```python
from build123d import *

# Parameters (mm, degrees)
F0_R     = 50.8
F1_DEPTH = 635
F2_W     = 50.8
F2_H     = 50.8
F3_DEPTH = 76.2
F4_R     = 19.05


with BuildPart() as f1:
    # F0 (on Top) → F1 (new body)
    with BuildSketch(Plane.XY):
        Circle(F0_R)
    extrude(amount=F1_DEPTH)

    # F2 (on face) → F3 (join)
    with BuildSketch(Plane.XY.offset(635)):
        Rectangle(F2_W, F2_H)
    extrude(amount=F3_DEPTH)

    # F4
    f4_edges = [f1.edges().sort_by_distance(p)[0] for p in [
        (25.4, -25.4, 673.1),
        (-25.4, -25.4, 673.1),
        (25.4, 25.4, 673.1),
        (-25.4, 25.4, 673.1),
    ]]
    fillet(f4_edges, radius=F4_R)


solid = f1.part
```
Geometry check sheet. Reference: the model listing, model coordinates, mm. A direction names the side the tool comes from. Give positions to 0.01 mm unless a question says otherwise; leave off trailing zeros. Order: outer loops, then holes, each group sorted by start corner. A loop starts at its lowest first (then second) coordinate and runs counter-clockwise, first axis right, second up. Notation, with made-up numbers: (-35, 50) -> (8, 50) arc R5 ccw to (8, 59) -> close; hole circle Ø11 at (-30.5, 22). An arc over 180 degrees is marked (long way). Write each question's results on one line, items separated by ' | '. Start each with the question number.
(1) Sectioned sample at A-A (y = 0). Enter the section's corners in (x, z).
(2) Sectioned sample at D-D (y = -38). Enter the section's corners in (x, z).
(3) Access from +Z, -Z, +X, -X, +Y, -Y to the whole of each face (thin tool, end or side, straight path). Record for faces 1 (the face through (-25.4, 0, 673)), 2 (the face through (22, -22, 635)), 3 (the face through (-19.67, 19.97, 673.63)), 4 (the face through (0, 25.4, 673)).
(4) Gauge pin test, flat ends, axial feed: P1, Ø6.5, axis at x = 0.5, z = 684.5, coming from the +Y side; P2, Ø12, axis at y = -25, z = 100.5, coming from the -X side; P3, Ø10, axis at y = -1.5, z = 669, coming from the +X side. Record the tip position at first contact, or that the pin passes through.
(5) Sectioned sample at C-C (z = 113). Enter the section's corners in (x, y).
(6) Scan lines: line 1 (X direction, y = -2, z = 596.5); line 2 (Z direction, x = -30, y = 27.5); line 3 (X direction, y = -9.5, z = 419). Record each from-to range of solid material in increasing order.
Answer below:
1) outline: (-50.8, 0) -> (50.8, 0) -> (50.8, 635) -> (25.4, 635) -> (25.4, 711.2) -> (-25.4, 711.2) -> (-25.4, 635) -> (-50.8, 635) -> close
2) outline: (-33.71, 0) -> (33.71, 0) -> (33.71, 635) -> (-33.71, 635) -> close
3) face 1: +Z, -X, +Y, -Y | face 2: +Z | face 3: +Z, -X, +Y | face 4: +Z, +X, -X, +Y
4) P1: y = 25.4 | P2: x = -47.11 | P3: x = 25.4
5) outline: circle Ø101.6 at (0, 0)
6) line 1: -50.76 to 50.76 | line 2: 0 to 635 | line 3: -49.9 to 49.9
